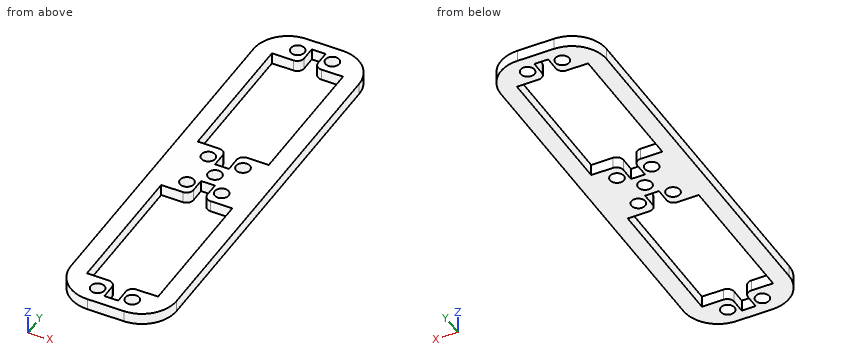
from build123d import *

# Parameters (mm, degrees)
SKETCH2_R           = 2
BOSS_EXTRUDE1_DEPTH = 1.65


with BuildPart() as part:
    # Sketch2 → Boss-Extrude1 (new body, symmetric)
    with BuildSketch(Plane.XY):
        with BuildLine():
            Line((-5.25, -60), (5.25, -60))
            ThreePointArc((5.25, -60), (12.321067812, -57.071067812), (15.25, -50))
            Line((15.25, -50), (15.25, 50))
            ThreePointArc((15.25, 50), (12.321067812, 57.071067812), (5.25, 60))
            Line((5.25, 60), (-5.25, 60))
            ThreePointArc((-5.25, 60), (-12.321067812, 57.071067812), (-15.25, 50))
            Line((-15.25, 50), (-15.25, -50))
            ThreePointArc((-15.25, -50), (-12.321067812, -57.071067812), (-5.25, -60))
        make_face()
        Circle(SKETCH2_R, mode=Mode.SUBTRACT)
        with Locations((5, 5.85)):
            Circle(SKETCH2_R, mode=Mode.SUBTRACT)
        with Locations((5, -5.85)):
            Circle(SKETCH2_R, mode=Mode.SUBTRACT)
        with Locations((-5, -5.85)):
            Circle(SKETCH2_R, mode=Mode.SUBTRACT)
        with Locations((-5, 5.85)):
            Circle(SKETCH2_R, mode=Mode.SUBTRACT)
        with Locations((5, 54.85)):
            Circle(SKETCH2_R, mode=Mode.SUBTRACT)
        with Locations((5, -54.85)):
            Circle(SKETCH2_R, mode=Mode.SUBTRACT)
        with Locations((-5, -54.85)):
            Circle(SKETCH2_R, mode=Mode.SUBTRACT)
        with Locations((-5, 54.85)):
            Circle(SKETCH2_R, mode=Mode.SUBTRACT)
        with BuildLine():
            Line((-10.25, 50.7), (-4, 50.7))
            ThreePointArc((-4, 50.7), (-2.585786438, 51.285786438), (-2, 52.7))
            Line((-2, 52.7), (-2, 56.85))
            Line((-2, 56.85), (2, 56.85))
            Line((2, 56.85), (2, 52.7))
            ThreePointArc((2, 52.7), (2.585786438, 51.285786438), (4, 50.7))
            Line((4, 50.7), (10.25, 50.7))
            Line((10.25, 50.7), (10.25, 10))
            Line((10.25, 10), (4, 10))
            ThreePointArc((4, 10), (2.585786438, 9.414213562), (2, 8))
            Line((2, 8), (2, 3.85))
            Line((2, 3.85), (-2, 3.85))
            Line((-2, 3.85), (-2, 8))
            ThreePointArc((-2, 8), (-2.585786438, 9.414213562), (-4, 10))
            Line((-4, 10), (-10.25, 10))
            Line((-10.25, 10), (-10.25, 50.7))
        make_face(mode=Mode.SUBTRACT)
        with BuildLine():
            Line((-10.25, -50.7), (-4, -50.7))
            ThreePointArc((-4, -50.7), (-2.585786438, -51.285786438), (-2, -52.7))
            Line((-2, -52.7), (-2, -56.85))
            Line((-2, -56.85), (2, -56.85))
            Line((2, -56.85), (2, -52.7))
            ThreePointArc((2, -52.7), (2.585786438, -51.285786438), (4, -50.7))
            Line((4, -50.7), (10.25, -50.7))
            Line((10.25, -50.7), (10.25, -10))
            Line((10.25, -10), (4, -10))
            ThreePointArc((4, -10), (2.585786438, -9.414213562), (2, -8))
            Line((2, -8), (2, -3.85))
            Line((2, -3.85), (-2, -3.85))
            Line((-2, -3.85), (-2, -8))
            ThreePointArc((-2, -8), (-2.585786438, -9.414213562), (-4, -10))
            Line((-4, -10), (-10.25, -10))
            Line((-10.25, -10), (-10.25, -50.7))
        make_face(mode=Mode.SUBTRACT)
    extrude(amount=BOSS_EXTRUDE1_DEPTH, both=True)


solid = part.part
The model under review builds one solid part; all positions refer to its coordinate system, in mm. Coordinates: 2 decimals unless noted, no trailing zeros. Loops run counter-clockwise (first coordinate to the right, second up) from the corner with the lowest first, then second, coordinate; pieces in that order, holes last. Notation, with made-up numbers: M 18.25,25.25 L 75.25,25.25 A15 cw 75.25,35.25 Z; hole C -4.5,-10.75 d5. An arc over 180 degrees is marked long. Put each result on its own line as item: value. Start each with the question number.
Q1. Wall thickness on line 1 (X direction, y = 13.5, z = -1.35); line 2 (Y direction, x = 0, z = 0.3); line 3 (Y direction, x = 8, z = 0.1): over which ranges is each line inside the solid? List them lowest first.
Q2. Add section A-A (y = 5.85). Write out the cut boundary in (x, z).
Q3. Add section D-D (y = 54.85). Write out the cut boundary in (x, z), and give its area (3 significant figures).
Q4. Add section B-B (y = -34). Write out the cut boundary in (x, z), and give its area (3 significant figures).
Q5. Clearance check with flat-ended pins moving along their axes: pin 1 (1 mm diameter, centred on x = -5.5, z = 0, fed in from -Y); pin 2 (1 mm diameter, centred on y = 54.5, z = 0.5, fed in from -X). State where each tip first meets the part, or that it passes through.
Q6. Add section C-C (z = -0.15). Count the separate pieces of the cut face and the enclosed holes in it, and give its area (3 significant figures).
Answers:
1. line 1: x = -15.25 to -10.25, 10.25 to 15.25
1. line 2: y = -60 to -56.85, -3.85 to -2, 2 to 3.85, 56.85 to 60
1. line 3: y = -59.61 to -50.7, -10 to 10, 50.7 to 59.61
2. outline: M -15.25,-1.65 L -7,-1.65 L -7,1.65 L -15.25,1.65 Z; M -3,-1.65 L -2,-1.65 L -2,1.65 L -3,1.65 Z; M 2,-1.65 L 3,-1.65 L 3,1.65 L 2,1.65 Z; M 7,-1.65 L 15.25,-1.65 L 15.25,1.65 L 7,1.65 Z
3. outline: M -14,-1.65 L -7,-1.65 L -7,1.65 L -14,1.65 Z; M -3,-1.65 L -2,-1.65 L -2,1.65 L -3,1.65 Z; M 2,-1.65 L 3,-1.65 L 3,1.65 L 2,1.65 Z; M 7,-1.65 L 14,-1.65 L 14,1.65 L 7,1.65 Z
3. area: 52.8 mm^2
4. outline: M -15.25,-1.65 L -10.25,-1.65 L -10.25,1.65 L -15.25,1.65 Z; M 10.25,-1.65 L 15.25,-1.65 L 15.25,1.65 L 10.25,1.65 Z
4. area: 33.0 mm^2
5. pin 1: stops at y = -60
5. pin 2: stops at x = -14.42
6. separate pieces: 1
6. enclosed holes: 11
6. area: 1,690 mm^2
